```python
from build123d import *

# Parameters (mm, degrees)
ESQUISSE2_R        = 3.96875
BOSS_EXTRU_6_DEPTH = 5
BOSS_EXTRU_7_DEPTH = 5
CONG_1_R           = 9
CONG_2_R           = 2.5


with BuildPart() as part:
    # Esquisse2 → Boss.-Extru.6 (new body)
    with BuildSketch(Plane.XY):
        Polygon((0, 0), (0, 90), (19.215728753, 109.215728753), (29.215728753, 109.215728753), (32.715728753, 105.715728753), (50.715728753, 105.715728753), (50.715728753, 87.715728753), (32.715728753, 87.715728753), (29.215728753, 84.215728753), (22.5, 84.215728753), (15, 76.715728753), (15, 0), align=None)
        with Locations((41.715728753, 96.715728753)):
            Circle(ESQUISSE2_R, mode=Mode.SUBTRACT)
    extrude(amount=BOSS_EXTRU_6_DEPTH)

    # Esquisse3 → Boss.-Extru.7 (add, through all)
    with BuildSketch(Plane.XY.offset(5)):
        with BuildLine():
            Line((38.666240834, 99.255728753), (44.765216671, 99.255728753))
            ThreePointArc((44.765216671, 99.255728753), (41.715728753, 100.684478753), (38.666240834, 99.255728753))
        make_face()
    extrude(amount=-BOSS_EXTRU_7_DEPTH)

    # Congé1
    cong_1_edges = [part.edges().sort_by_distance(p)[0] for p in [
        (50.715728753, 87.715728753, 2.5),
        (50.715728753, 105.715728753, 2.5),
    ]]
    fillet(cong_1_edges, radius=CONG_1_R - 0.0001)  # a hair under: the kernel refuses the full size

    # Congé2
    cong_2_edges = [part.edges().sort_by_distance(p)[0] for p in [
        (0, 90, 2.5),
        (19.215728753, 109.215728753, 2.5),
        (29.215728753, 109.215728753, 2.5),
        (32.715728753, 105.715728753, 2.5),
        (32.715728753, 87.715728753, 2.5),
        (29.215728753, 84.215728753, 2.5),
        (22.5, 84.215728753, 2.5),
        (15, 76.715728753, 2.5),
    ]]
    fillet(cong_2_edges, radius=CONG_2_R)


solid = part.part
```
For this review, take the finished solid that the model builds, in its own axes (mm). A direction names the side the tool comes from. Round coordinates to 2 decimals unless told otherwise and drop trailing zeros. Write each loop counter-clockwise with the first axis right and the second up, starting at its lowest first coordinate (ties: lowest second). Pieces come first, ordered by that corner, then holes.
1) Mouldability with a two-part tool opening along Y and no side actions: class faces 1 (the face through (38, 105.716, 2)), 2 (the face through (42, 99.256, 3)), 3 (the face through (8, 0, 2)), 4 (the face through (41.59, 92.75, 2.46)) as +Y half, -Y half, draft (parallel to the pull), parting line (faces both ways), or undercut.
Answer below:
face 1: +Y half
face 2: undercut
face 3: -Y half
face 4: undercut
2) Take a section at C-C on x = 6.5. Give the boundary of the cut face in (y, z).
Answer below:
outline: (0, 0) - (96.5, 0) - (96.5, 5) - (0, 5) - close
3) Machinability: for faces 5 (the face through (14, 68, 5)), 6 (the face through (38, 87.716, 2)), which of the approach directions +Z, -Z, +X, -X, +Y, -Y give a long, thin tool a straight path to every point of the face, cutting with its end or side? Answer none if there is none.
Answer below:
face 5: +Z, +X, -X, +Y, -Y
face 6: +Z, -Z, +X, -Y
4) For line 1 along X through (y, z) = (67.5, 1); line 2 along Y through (x, z) = (3, 1.9); line 3 along Y through (x, z) = (26, 0.4), list the stretches that pass through material, from the lowest coordinate up.
Answer below:
line 1: x = 0 to 15
line 2: y = 0 to 93
line 3: y = 84.22 to 109.22
5) Insertion check: pin 1 Ø2.5 at (y, z) = (24, 3.5) entering from +X; pin 2 Ø1.4 at (x, z) = (25, 2) entering from -Y; pin 3 Ø1.5 at (x, z) = (43, 2) entering from -Y. Each pin has a flat end and moves straight along its axis. Give the tip position at first contact, or say it passes through.
Answer below:
pin 1: stops at x = 15
pin 2: stops at y = 84.22
pin 3: stops at y = 87.73
6) Take a section at B-B on y = 11. Give the boundary of the cut face in (x, z).
Answer below:
outline: (0, 0) - (15, 0) - (15, 5) - (0, 5) - close
